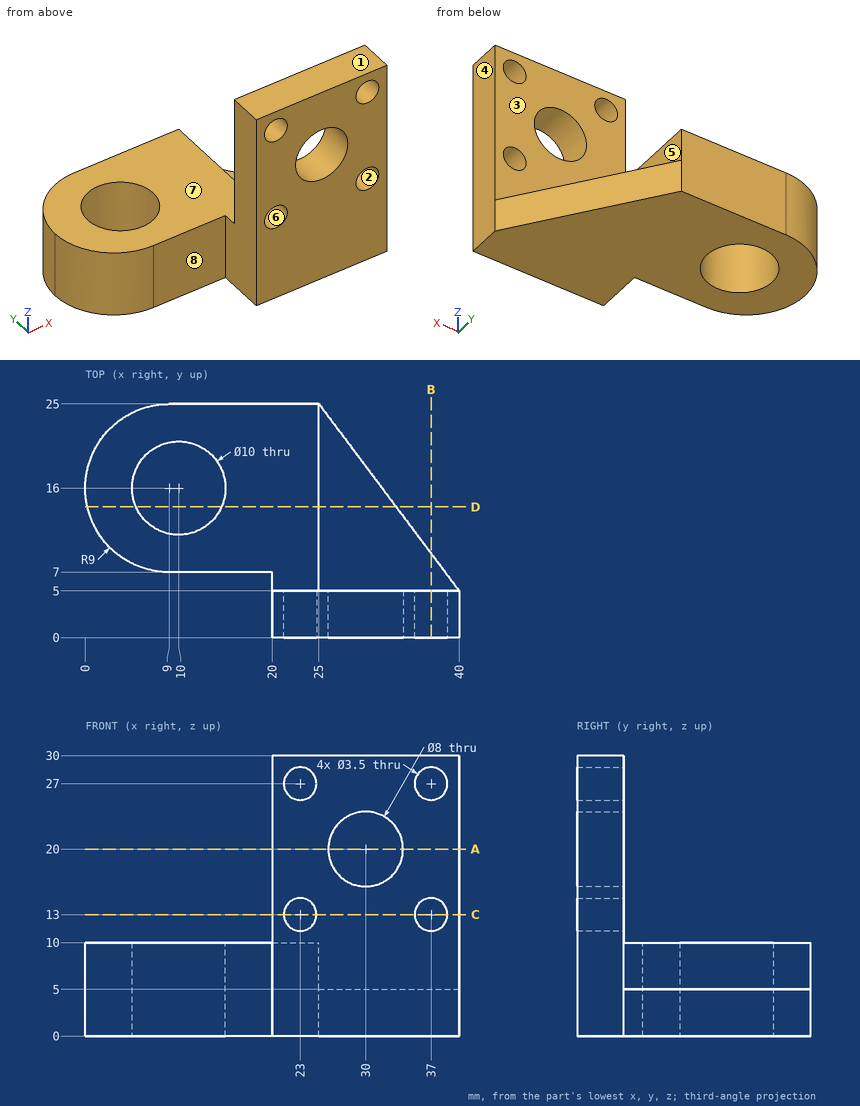
Geometry: see drawing. Coordinates: mm, zero at the bounding-box minimum. A direction names the side the tool comes from. Coordinates: 2 decimals unless noted, no trailing zeros. Loops run counter-clockwise (first coordinate to the right, second up) from the corner with the lowest first, then second, coordinate; pieces in that order, holes last. Notation, with made-up numbers: (87.5, 22.5) -> (111.5, 22.5) arc R31 cw to (111.5, 59.5) -> close; hole circle Ø5 at (-21.75, 80). An arc over 180 degrees is marked (long way). Write item = value, one per line. Start each with the question number.
Item 1: Cut plane C-C, the plane z = 13. Return loops of the section in (x, y).
Item 2: First-contact query: P1, Ø4, axis at x = 23, z = 13, coming from the -Y side; P2, Ø3, axis at x = 24, z = 18.5, coming from the +Y side; P3, Ø11, axis at x = 13, z = 6, coming from the -Y side; P4, Ø7.5, axis at x = 32.5, y = 11, coming from the +Z side. Flat tips, straight axial feed; report the tip coordinate or a pass-through.
Item 3: Cut plane D-D, the plane y = 14. Return loops of the section in (x, z).
Item 4: Material intervals for line 1 (Z direction, x = 23, y = 2.85); line 2 (Y direction, x = 10, z = 6.5); line 3 (X direction, y = 16, z = 5.5), sorted ascending.
Item 5: Mould query, pull axis Z, two halves, no side actions, for the marked faces 1, 2 and 3. Classes: pulls with the +Z half, pulls with the -Z half, needs draft (parallel to the pull), parting line crosses it, or undercut.
Item 6: Reachability of the marked faces 4, 5, 6, 7 and 8 from +Z, -Z, +X, -X, +Y, -Y: full face, straight path, thin tool, end or side. Return the list, or none.
Item 7: Cut plane B-B, the plane x = 37. Return loops of the section in (y, z).
Item 8: Cut plane A-A, the plane z = 20. Return loops of the section in (x, y), plus the area to 3 significant figures.
Ans:
q1.outline = (20, 0) -> (21.25, 0) -> (21.25, 5) -> (20, 5) -> close; (24.75, 0) -> (35.25, 0) -> (35.25, 5) -> (24.75, 5) -> close; (38.75, 0) -> (40, 0) -> (40, 5) -> (38.75, 5) -> close
q2.P1 = 0
q2.P2 = 5
q2.P3 = 7
q2.P4 = 5
q3.outline = (0.23, 0) -> (5.42, 0) -> (5.42, 10) -> (0.23, 10) -> close; (14.58, 0) -> (33.25, 0) -> (33.25, 5) -> (25, 5) -> (25, 10) -> (14.58, 10) -> close
q4.line_1 = 0 to 11.25, 14.75 to 25.25, 28.75 to 30
q4.line_2 = 7 to 11, 21 to 25
q4.line_3 = 0 to 5, 15 to 25
q5.face_1 = pulls with the +Z half
q5.face_2 = undercut
q5.face_3 = needs draft
q6.face_4 = +Z, -Z, +X, +Y, -Y
q6.face_5 = +Z, +X, +Y
q6.face_6 = +Y, -Y
q6.face_7 = +Z, +X, -X, +Y
q6.face_8 = +Z, -Z, -X, -Y
q7.outline = (0, 0) -> (9, 0) -> (9, 5) -> (5, 5) -> (5, 11.25) -> (0, 11.25) -> close; (0, 14.75) -> (5, 14.75) -> (5, 25.25) -> (0, 25.25) -> close; (0, 28.75) -> (5, 28.75) -> (5, 30) -> (0, 30) -> close
q8.outline = (20, 0) -> (26, 0) -> (26, 5) -> (20, 5) -> close; (34, 0) -> (40, 0) -> (40, 5) -> (34, 5) -> close
q8.area = 60.0 mm²
